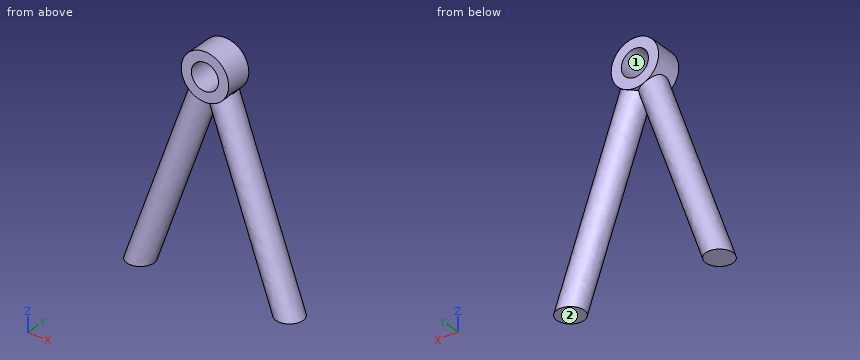
from build123d import *

# Parameters (mm, degrees)
F0_R     = 10
F4_R     = 17.5
F4_R_2   = 10
F5_DEPTH = 10


with BuildPart() as f2:
    # F2: sweep along a path in F1
    with BuildLine(Plane.XZ) as f2_path:
        Line((-55, 0), (-5, 140))
    # F0 (on Top) → F2 (sweep)
    with BuildSketch(Plane.XY):
        with Locations((-55, 0)):
            Circle(F0_R)
    sweep(path=f2_path.line)

    # F3: sweep along a path in F1
    with BuildLine(Plane.XZ) as f3_path:
        Line((55, 0), (5, 140))
    # F0 (on Top) → F3 (sweep)
    with BuildSketch(Plane.XY):
        with Locations((55, 0)):
            Circle(F0_R)
    sweep(path=f3_path.line)

    # F4 (on Front) → F5 (join, symmetric)
    with BuildSketch(Plane.XZ):
        with Locations((0, 150)):
            Circle(F4_R)
        with Locations((0, 150)):
            Circle(F4_R_2, mode=Mode.SUBTRACT)
    extrude(amount=F5_DEPTH, both=True)


solid = f2.part
Input: part model. Units: mm. Frame: model coordinates. Face numbers are marked on the shaded views. Coordinates: 2 decimals unless noted, no trailing zeros. Loops run counter-clockwise (first coordinate to the right, second up) from the corner with the lowest first, then second, coordinate; pieces in that order, holes last.
Q1. Contact query for flat-ended pins moving along their axis: pin 1 (5 mm diameter, centred on y = 4.5, z = 46.5, fed in from +X); pin 2 (1.5 mm diameter, centred on y = 7.5, z = 60.5, fed in from -X); pin 3 (4 mm diameter, centred on y = 7.5, z = 59.5, fed in from -X). Output: stop coordinate, or through.
Q2. Material intervals for line 1 (X direction, y = -2, z = 25.5); line 2 (X direction, y = 7.25, z = 93); line 3 (Y direction, x = 46.5, z = 7.5), sorted ascending.
Q3. Draft query along X for the marked faces 1 and 2. Return one class per face: +X half, -X half, draft (parallel to the pull), parting line (faces both ways), or undercut.
Q4. Cut plane A-A (z = 150). Output: boundary loops of the cut face in (x, y), then the cut area to 3 significant figures.
Working result:
1. pin 1: stops at x = 48.65
1. pin 2: stops at x = -40.82
1. pin 3: stops at x = -42.28
2. line 1: x = -55.69 to -36.09, 36.09 to 55.69
2. line 2: x = -28.67 to -14.9, 14.9 to 28.67
2. line 3: y = -8.13 to 8.13
3. face 1: undercut
3. face 2: draft
4. outline: (-17.5, -10) - (-10, -10) - (-10, 10) - (-17.5, 10) - close; (10, -10) - (17.5, -10) - (17.5, 10) - (10, 10) - close
4. area: 300 mm2
